Build history of the part. All positions in model axes, mm. Give positions to 0.01 mm unless a question says otherwise; leave off trailing zeros. Use a Markdown table: item, result. Add a question column.
(1) Wall check: line 1 (Z direction, x = -6, y = 0.15); line 2 (Z direction, x = 12.5, y = 0.5); line 3 (Z direction, x = 0, y = 0.25). Give the ranges that are in metal, low to high.
(2) Flat gauge pin, fed straight in: pin 1 (12 mm diameter, centred on x = 5.5, z = 9, fed in from +Y). Where does the tip first touch, or does it go through?
(3) Slice it at A-A (y = 0.1). Count the separate pieces of the cut face and the enclosed holes in it, then the cut area to 3 significant figures.
from build123d import *

# Parameters (mm, degrees)
SKETCH1_R                    = 17.5
BOSS_EXTRUDE1_DEPTH          = 0.6
CUT_EXTRUDE1_REACH           = 2.6
SKETCH2_R                    = 13.5
SKETCH3_R                    = 1.6
CUT_EXTRUDE2_DEPTH           = 0.6
CIRPATTERN1_COUNT            = 6
CIRPATTERN1_ANGLE            = 100
SKETCH4_R                    = 1.6
CUT_EXTRUDE3_DEPTH           = 0.6
CIRPATTERN2_COUNT            = 11
CIRPATTERN2_ANGLE            = 200
F_1_0_1_DIAMETER_HOLE1_D     = 1
F_1_0_1_DIAMETER_HOLE1_DEPTH = 0.6
CHAMFER1_SIZE                = 0.2


with BuildPart() as part:
    # Sketch1 → Boss-Extrude1 (new body)
    with BuildSketch(Plane(origin=(0, 0, 0), x_dir=(1, 0, 0), z_dir=(0, 1, 0))):
        Circle(SKETCH1_R)
    extrude(amount=BOSS_EXTRUDE1_DEPTH)

    # Sketch2 → Cut-Extrude1 (cut, up to next)
    with BuildSketch(Plane(origin=(0, 0.6, 0), x_dir=(1, 0, 0), z_dir=(0, 1, 0)), mode=Mode.PRIVATE) as cut_extrude1_sk1:
        Circle(SKETCH2_R)
    cut_extrude1_tool1 = extrude(cut_extrude1_sk1.sketch, amount=-CUT_EXTRUDE1_REACH, mode=Mode.PRIVATE) & part.part
    add(cut_extrude1_tool1.solids().sort_by_distance((0, 0.6, 0))[0], mode=Mode.SUBTRACT)

    # Sketch3 → Cut-Extrude2 (cut)
    with BuildSketch(Plane(origin=(0, 0.6, 0), x_dir=(1, 0, 0), z_dir=(0, 1, 0))):
        with Locations((11.691342951, 6.75)):
            Circle(SKETCH3_R)
    cut_extrude2 = extrude(amount=-CUT_EXTRUDE2_DEPTH, mode=Mode.SUBTRACT)

    # CirPattern1: Cut-Extrude2 ×6 about axis
    cirpattern1_axis = Axis((0, 0, 0), (0, 1, 0))
    for i in range(1, CIRPATTERN1_COUNT):
        add(cut_extrude2.rotate(cirpattern1_axis, i * CIRPATTERN1_ANGLE / (CIRPATTERN1_COUNT - 1)), mode=Mode.SUBTRACT)

    # Sketch4 → Cut-Extrude3 (cut)
    with BuildSketch(Plane(origin=(0, 0.6, 0), x_dir=(1, 0, 0), z_dir=(0, 1, 0))):
        with Locations((13.5, 0)):
            Circle(SKETCH4_R)
    cut_extrude3 = extrude(amount=-CUT_EXTRUDE3_DEPTH, mode=Mode.SUBTRACT)

    # CirPattern2: Cut-Extrude3 ×11 about axis
    cirpattern2_axis = Axis((0, 0, 0), (0, -1, 0))
    for i in range(1, CIRPATTERN2_COUNT):
        add(cut_extrude3.rotate(cirpattern2_axis, i * CIRPATTERN2_ANGLE / (CIRPATTERN2_COUNT - 1)), mode=Mode.SUBTRACT)

    # Ø1.0 (1) Diameter Hole1
    with Locations(Plane(origin=(0, 0.6, 0), x_dir=(1, 0, 0), z_dir=(0, 1, 0))):
        with Locations((15.841183551, 4.24463234), (-13.434093526, 9.406653556), (-5.609130351, -15.410958981)):
            Hole(F_1_0_1_DIAMETER_HOLE1_D / 2, depth=F_1_0_1_DIAMETER_HOLE1_DEPTH)

    # Chamfer1
    chamfer1_edges = [part.edges().sort_by_distance(p)[0] for p in [
        (-17.5, 0, 0),
    ]]
    chamfer(chamfer1_edges, length=CHAMFER1_SIZE)


solid = part.part
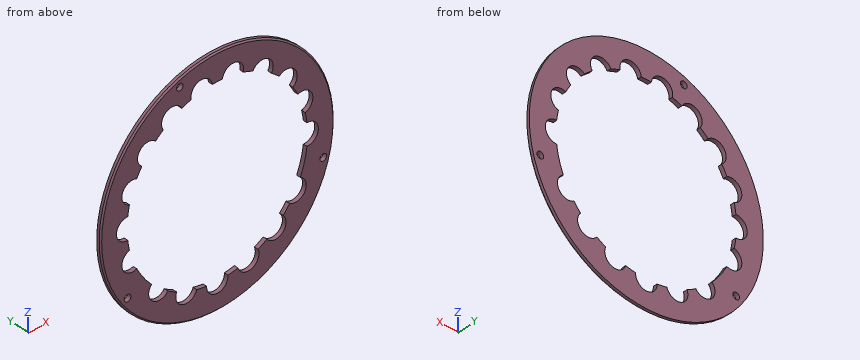
Solution:
| question | item | result |
|---|---|---|
| 1 | line 1 | -16.39 to -13.49, 13.1 to 15.1, 15.72 to 16.39 |
| 1 | line 2 | -12.25 to -8.13, -5.37 to -5.1, 6.21 to 12.25 |
| 1 | line 3 | -17.5 to -15.1, 13.5 to 17.5 |
| 2 | pin 1 | y = 0.6 |
| 3 | separate pieces | 1 |
| 3 | enclosed holes | 4 |
| 3 | area | 306 mm2 |
